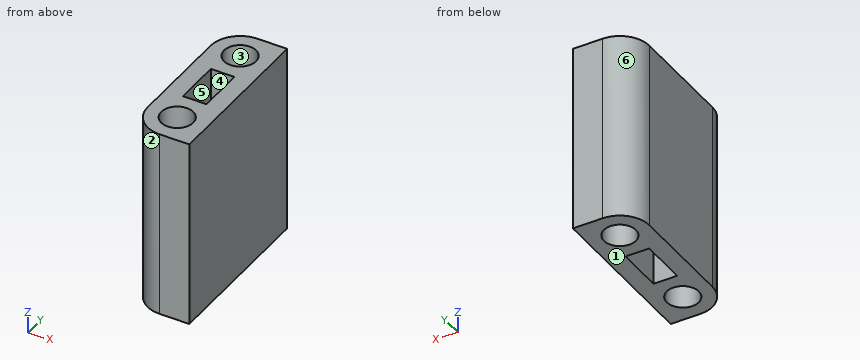
from build123d import *

# Parameters (mm, degrees)
F0_W     = 7.9375
F0_H     = 22.225
F0_W_2   = 3.175
F0_H_2   = 6.35
F1_DEPTH = 25.4
F2_R     = 2.15265
F3_DEPTH = 25.4
F4_R     = 3.96875


with BuildPart() as f1:
    # F0 (on Top) → F1 (new body)
    with BuildSketch(Plane.XY):
        Rectangle(F0_W, F0_H)
        Rectangle(F0_W_2, F0_H_2, mode=Mode.SUBTRACT)
    extrude(amount=F1_DEPTH)

    # F2 (on face) → F3 (cut, through all)
    with BuildSketch(Plane.XY.offset(25.4)):
        with Locations((0, 7.14375)):
            Circle(F2_R)
        with Locations((0, -7.14375)):
            Circle(F2_R)
    extrude(amount=-F3_DEPTH, mode=Mode.SUBTRACT)

    # F4
    f4_edges = [f1.edges().sort_by_distance(p)[0] for p in [
        (-3.96875, -11.1125, 12.7),
        (-3.96875, 11.1125, 12.7),
    ]]
    fillet(f4_edges, radius=F4_R)


solid = f1.part
Build history of the part. All positions in model axes, mm. Face numbers are marked on the shaded views. A direction names the side the tool comes from. Round coordinates to 2 decimals unless told otherwise and drop trailing zeros. Loops run counter-clockwise (first coordinate to the right, second up) from the corner with the lowest first, then second, coordinate; pieces in that order, holes last. Notation, with made-up numbers: (-15, 70.25) -> (19, 70.25) arc R6 cw to (19, 81.25) -> close; hole circle Ø9 at (59, 66.5). An arc over 180 degrees is marked (long way). Answer in a Markdown table with one row per item.
Item 1: Which spindle directions (+Z, -Z, +X, -X, +Y, -Y) get a long thin tool onto all of the face, cutting with end or side? Do the marked faces 5 and 6. Say none if no direction does.
Answers below:
| item | result |
|---|---|
| face 5 | +Z, -Z |
| face 6 | +Z, -Z, -X, +Y |
Item 2: Drill centre lines: L1, parallel to Y at x = 0, z = 11 (1 decimal); L2, parallel to X at y = -2.5, z = 5.25; L3, parallel to Y at x = 1, z = 2 (1 decimal). Where is each one in solid material? Low to high. Write a range as [from, to].
Answers below:
| item | result |
|---|---|
| L1 | y = [-11.1, -9.3], [-5, -3.2], [3.2, 5], [9.3, 11.1] |
| L2 | x = [-3.97, -1.59], [1.59, 3.97] |
| L3 | y = [-11.1, -9.1], [-5.2, -3.2], [3.2, 5.2], [9.1, 11.1] |
Item 3: Mould opens along Y. For the marked faces 1, 2, 3 and 4 say: +Y half, -Y half, draft (parallel to the pull), parting line (faces both ways), or undercut.
Answers below:
| item | result |
|---|---|
| face 1 | draft |
| face 2 | -Y half |
| face 3 | undercut |
| face 4 | undercut |
Item 4: Saw through at B-B (z = 19.75). Write the cut outline in (x, y) (1 decimal).
Answers below:
| item | result |
|---|---|
| outline | (-4, -7.1) arc R4 ccw to (0, -11.1) -> (4, -11.1) -> (4, 11.1) -> (0, 11.1) arc R4 ccw to (-4, 7.1) -> close; hole circle Ø4.3 at (0, -7.1); hole circle Ø4.3 at (0, 7.1); hole (-1.6, -3.2) -> (1.6, -3.2) -> (1.6, 3.2) -> (-1.6, 3.2) -> close |
Item 5: Saw through at A-A (y = -2). Write the cut outline in (x, z).
Answers below:
| item | result |
|---|---|
| outline | (-3.97, 0) -> (-1.59, 0) -> (-1.59, 25.4) -> (-3.97, 25.4) -> close; (1.59, 0) -> (3.97, 0) -> (3.97, 25.4) -> (1.59, 25.4) -> close |
